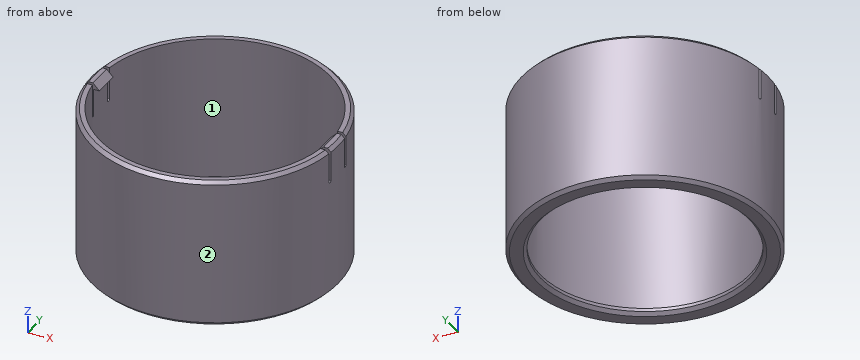
from build123d import *

# Parameters (mm, degrees)
F0_R          = 18.875
F0_R_2        = 17.625
F1_DEPTH      = 23
F0_R_3        = 16
F2_DEPTH      = 1
F3_SIZE       = 0.5
F5_DEPTH      = 25
F5_DEPTH_BACK = 25
F7_DEPTH      = 1
F8_SIZE       = 0.99999


# Not quite as in the source:
# - a fillet or chamfer is up to 0.001 mm smaller than in the source, because OpenCascade refuses the exact size


with BuildPart() as f1:
    # F0 (on Top) → F1 (new body)
    with BuildSketch(Plane.XY):
        Circle(F0_R)
        Circle(F0_R_2, mode=Mode.SUBTRACT)
    extrude(amount=F1_DEPTH)

    # F0 (on Top) → F2 (join)
    with BuildSketch(Plane.XY):
        Circle(F0_R_2)
        Circle(F0_R_3, mode=Mode.SUBTRACT)
    extrude(amount=F2_DEPTH)

    # F3
    f3_edges = [f1.edges().sort_by_distance(p)[0] for p in [
        (-18.875, 0, 0),
        (-16, 0, 0),
        (-18.875, 0, 23),
    ]]
    chamfer(f3_edges, length=F3_SIZE)

    # F4 (on Right) → F5 (cut, two sides)
    with BuildSketch(Plane.YZ) as f5_sk:
        with BuildLine():
            Line((-2.5, 18), (-2, 18))
            ThreePointArc((-2, 18), (-2.25, 18.25), (-2.5, 18))
        make_face()
        with BuildLine():
            ThreePointArc((-2.5, 18), (-2.25, 17.75), (-2, 18))
            Line((-2, 18), (-2.5, 18))
        make_face()
        with BuildLine():
            ThreePointArc((-2.5, 18), (-2.25, 18.25), (-2, 18))
            Line((-2, 18), (-2, 23))
            Line((-2, 23), (-2.5, 23))
            Line((-2.5, 23), (-2.5, 18))
        make_face()
        with BuildLine():
            Line((2.5, 23), (2, 23))
            Line((2, 23), (2, 18))
            ThreePointArc((2, 18), (2.25, 18.25), (2.5, 18))
            Line((2.5, 18), (2.5, 23))
        make_face()
        with BuildLine():
            ThreePointArc((2.5, 18), (2.25, 18.25), (2, 18))
            Line((2, 18), (2.5, 18))
        make_face()
        with BuildLine():
            Line((2.5, 18), (2, 18))
            ThreePointArc((2, 18), (2.25, 17.75), (2.5, 18))
        make_face()
    extrude(amount=-F5_DEPTH, mode=Mode.SUBTRACT)
    extrude(f5_sk.sketch, amount=F5_DEPTH_BACK, mode=Mode.SUBTRACT)

    # F6 (on face) → F7 (join)
    with BuildSketch(Plane.XY.offset(23)):
        with BuildLine():
            ThreePointArc((-17.5111571577, 2), (-17.5965162732, 1.001618714), (-17.625, 0))
            Line((-17.625, 0), (-16.625, 0))
            Line((-16.625, 0), (-16.625, 2))
            Line((-16.625, 2), (-17.5111571577, 2))
        make_face()
        with BuildLine():
            Line((-16.625, 0), (-17.625, 0))
            ThreePointArc((-17.625, 0), (-17.5965162732, -1.001618714), (-17.5111571577, -2))
            Line((-17.5111571577, -2), (-16.625, -2))
            Line((-16.625, -2), (-16.625, 0))
        make_face()
        Polygon((17.8884946657, 2), (17.5111571577, 2), (16.625, 2), (16.625, 0), (16.625, -2), (17.8884946657, -2), align=None)
    extrude(amount=-F7_DEPTH)

    # F8 (size 1 in the source; OpenCascade refuses exactly that, so slightly less here)
    f8_edges = [f1.edges().sort_by_distance(p)[0] for p in [
        (-16.625, 0, 23),
        (16.625, 0, 23),
    ]]
    chamfer(f8_edges, length=F8_SIZE)


solid = f1.part
Build history of the part. All positions in model axes, mm. Face numbers are marked on the shaded views. Coordinates: 2 decimals unless noted, no trailing zeros. Write each loop counter-clockwise with the first axis right and the second up, starting at its lowest first coordinate (ties: lowest second). Pieces come first, ordered by that corner, then holes. Notation, with made-up numbers: (30.25, 8) -> (46.25, 8) arc R30 ccw to (46.25, 32) -> close; hole circle Ø10 at (-15.75, 23.5). An arc over 180 degrees is marked (long way). Use CSV: the item, a comma, the result in double quotes. Start each with the question number.
Q1. Pull direction Y, two halves, no side cores. Call the marked faces 1 and 2: released by +Y, released by -Y, zero draft, split by the parting line, or undercut.
Q2. Cut at C-C, the plane z = 4. List the corners of the cut face in (x, y) (3 decimals), then the cut area to 3 significant figures.
Q3. Flat gauge pins, fed straight in: pin 1 Ø4 at (x, z) = (13.5, 9) entering from -Y; pin 2 Ø2.5 at (x, z) = (18, 21.5) entering from +Y; pin 3 Ø8 at (x, z) = (9.5, 4) entering from +Y. Where does each tip first touch, or does it go through?
Q4. Cut at B-B, the plane z = 21.5. List the corners of the cut face in (x, y) (3 decimals).
Q5. Drill centre lines: probe 1 along Y at (x, z) = (0, 13) (3 decimals); probe 2 along X at (y, z) = (-2.5, 9.25); probe 3 along Y at (x, z) = (-4.5, 20.5). Where is each one in solid material? Low to high.
Checked values:
1,face 1,"undercut"
1,face 2,"split by the parting line"
2,outline,"circle Ø37.75 at (0, 0); hole circle Ø35.25 at (0, 0)"
2,area,"143 mm²"
3,pin 1,"stops at y = -14.97"
3,pin 2,"stops at y = 8.7"
3,pin 3,"stops at y = 18.06"
4,outline,"(-18.769, -2) -> (-17.511, -2) arc R17.625 cw to (-17.511, 2) -> (-18.769, 2) arc R18.875 ccw to start; (-18.709, -2.5) arc R18.875 ccw to (18.709, -2.5) -> (17.447, -2.5) arc R17.625 cw to (-17.447, -2.5) -> close; (-18.709, 2.5) -> (-17.447, 2.5) arc R17.625 cw to (17.447, 2.5) -> (18.709, 2.5) arc R18.875 ccw to start; (17.511, -2) -> (18.769, -2) arc R18.875 ccw to (18.769, 2) -> (17.511, 2) arc R17.625 cw to start"
5,probe 1,"y = -18.875 to -17.625, 17.625 to 18.875"
5,probe 2,"x = -18.71 to -17.45, 17.45 to 18.71"
5,probe 3,"y = -18.33 to -17.04, 17.04 to 18.33"
